```python
from build123d import *

# Parameters (mm, degrees)
BOSS_EXTRUDE1_DEPTH = 1
SKETCH3_W           = 55.6
SKETCH3_H           = 0.9
BOSS_EXTRUDE2_DEPTH = 3.24
FILLET1_R           = 1.5
FILLET2_R           = 1.5
FILLET3_R           = 1.5
FILLET4_R           = 1.5
CUT_EXTRUDE2_REACH  = 3
SKETCH5_R           = 1.6


with BuildPart() as part:
    # Sketch1 → Boss-Extrude1 (new body)
    with BuildSketch(Plane(origin=(0, 0, 0), x_dir=(1, 0, 0), z_dir=(0, 1, 0))):
        with BuildLine():
            Line((27.8, -18.75), (-27.8, -18.75))
            ThreePointArc((-27.8, -18.75), (-32.396194078, -16.846194078), (-34.3, -12.25))
            Line((-34.3, -12.25), (-34.3, 12.25))
            ThreePointArc((-34.3, 12.25), (-32.396194078, 16.846194078), (-27.8, 18.75))
            Line((-27.8, 18.75), (27.8, 18.75))
            ThreePointArc((27.8, 18.75), (32.396194078, 16.846194078), (34.3, 12.25))
            Line((34.3, 12.25), (34.3, -12.25))
            ThreePointArc((34.3, -12.25), (32.396194078, -16.846194078), (27.8, -18.75))
        make_face()
    extrude(amount=BOSS_EXTRUDE1_DEPTH)

    # Sketch3 → Boss-Extrude2 (add)
    with BuildSketch(Plane(origin=(0, 1, 0), x_dir=(1, 0, 0), z_dir=(0, 1, 0))):
        with Locations((0, -18.3)):
            Rectangle(SKETCH3_W, SKETCH3_H)
        with Locations((0, 18.3)):
            Rectangle(SKETCH3_W, SKETCH3_H)
    extrude(amount=BOSS_EXTRUDE2_DEPTH)

    # Fillet1
    fillet1_edges = [part.edges().sort_by_distance(p)[0] for p in [
        (-27.8, 4.24, 18.3),
    ]]
    fillet(fillet1_edges, radius=FILLET1_R)

    # Fillet2
    fillet2_edges = [part.edges().sort_by_distance(p)[0] for p in [
        (27.8, 4.24, 18.3),
    ]]
    fillet(fillet2_edges, radius=FILLET2_R)

    # Fillet3
    fillet3_edges = [part.edges().sort_by_distance(p)[0] for p in [
        (27.8, 4.24, -18.3),
    ]]
    fillet(fillet3_edges, radius=FILLET3_R)

    # Fillet4
    fillet4_edges = [part.edges().sort_by_distance(p)[0] for p in [
        (-27.8, 4.24, -18.3),
    ]]
    fillet(fillet4_edges, radius=FILLET4_R)

    # Sketch5 → Cut-Extrude2 (cut, up to next)
    with BuildSketch(Plane(origin=(0, 1, 0), x_dir=(1, 0, 0), z_dir=(0, 1, 0)), mode=Mode.PRIVATE) as cut_extrude2_sk1:
        with Locations((-25.4, -9.4746)):
            Circle(SKETCH5_R)
    cut_extrude2_tool1 = extrude(cut_extrude2_sk1.sketch, amount=-CUT_EXTRUDE2_REACH, mode=Mode.PRIVATE) & part.part
    add(cut_extrude2_tool1.solids().sort_by_distance((-25.4, 1, 9.4746))[0], mode=Mode.SUBTRACT)
    # Sketch5 → Cut-Extrude2 (cut, up to next)
    with BuildSketch(Plane(origin=(0, 1, 0), x_dir=(1, 0, 0), z_dir=(0, 1, 0)), mode=Mode.PRIVATE) as cut_extrude2_sk2:
        with Locations((-15.24, -9.4746)):
            Circle(SKETCH5_R)
    cut_extrude2_tool2 = extrude(cut_extrude2_sk2.sketch, amount=-CUT_EXTRUDE2_REACH, mode=Mode.PRIVATE) & part.part
    add(cut_extrude2_tool2.solids().sort_by_distance((-15.24, 1, 9.4746))[0], mode=Mode.SUBTRACT)
    # Sketch5 → Cut-Extrude2 (cut, up to next)
    with BuildSketch(Plane(origin=(0, 1, 0), x_dir=(1, 0, 0), z_dir=(0, 1, 0)), mode=Mode.PRIVATE) as cut_extrude2_sk3:
        with Locations((-5.08, -9.4746)):
            Circle(SKETCH5_R)
    cut_extrude2_tool3 = extrude(cut_extrude2_sk3.sketch, amount=-CUT_EXTRUDE2_REACH, mode=Mode.PRIVATE) & part.part
    add(cut_extrude2_tool3.solids().sort_by_distance((-5.08, 1, 9.4746))[0], mode=Mode.SUBTRACT)
    # Sketch5 → Cut-Extrude2 (cut, up to next)
    with BuildSketch(Plane(origin=(0, 1, 0), x_dir=(1, 0, 0), z_dir=(0, 1, 0)), mode=Mode.PRIVATE) as cut_extrude2_sk4:
        with Locations((5.08, -9.4746)):
            Circle(SKETCH5_R)
    cut_extrude2_tool4 = extrude(cut_extrude2_sk4.sketch, amount=-CUT_EXTRUDE2_REACH, mode=Mode.PRIVATE) & part.part
    add(cut_extrude2_tool4.solids().sort_by_distance((5.08, 1, 9.4746))[0], mode=Mode.SUBTRACT)
    # Sketch5 → Cut-Extrude2 (cut, up to next)
    with BuildSketch(Plane(origin=(0, 1, 0), x_dir=(1, 0, 0), z_dir=(0, 1, 0)), mode=Mode.PRIVATE) as cut_extrude2_sk5:
        with Locations((15.24, -9.4746)):
            Circle(SKETCH5_R)
    cut_extrude2_tool5 = extrude(cut_extrude2_sk5.sketch, amount=-CUT_EXTRUDE2_REACH, mode=Mode.PRIVATE) & part.part
    add(cut_extrude2_tool5.solids().sort_by_distance((15.24, 1, 9.4746))[0], mode=Mode.SUBTRACT)
    # Sketch5 → Cut-Extrude2 (cut, up to next)
    with BuildSketch(Plane(origin=(0, 1, 0), x_dir=(1, 0, 0), z_dir=(0, 1, 0)), mode=Mode.PRIVATE) as cut_extrude2_sk6:
        with Locations((25.4, -9.4746)):
            Circle(SKETCH5_R)
    cut_extrude2_tool6 = extrude(cut_extrude2_sk6.sketch, amount=-CUT_EXTRUDE2_REACH, mode=Mode.PRIVATE) & part.part
    add(cut_extrude2_tool6.solids().sort_by_distance((25.4, 1, 9.4746))[0], mode=Mode.SUBTRACT)


solid = part.part
```
Part model, mm, in its own coordinate system. A direction names the side the tool comes from. Round coordinates to 2 decimals unless told otherwise and drop trailing zeros. Loops run counter-clockwise (first coordinate to the right, second up) from the corner with the lowest first, then second, coordinate; pieces in that order, holes last.
Item 1: Cut at A-A, the plane x = 15.24. Give the cut face in (y, z), then the cut area to 3 significant figures.
Item 2: 3-axis set-ups, long thin cutter, end or side, ignore diameter. For faces 4 (the face through (0, 3, -17.85)), 5 (the face through (27.37, 3.79, -18.31)): which of +Z, -Z, +X, -X, +Y, -Y reach the whole face in a straight line?
Item 3: Cut at C-C, the plane z = 16. Give the cut face in (x, y).
Item 4: Mould opens along X. For faces 1 (the face through (27.35, 3.81, 18.29)), 2 (the face through (-15.587, 0.507, 11.037)), 3 (the face through (-27.37, 3.79, 18.29)) say: +X half, -X half, draft (parallel to the pull), parting line (faces both ways), or undercut.
Item 5: Drop flat-ended pins along their axis: P1, Ø0.7, axis at y = 2, z = -18, coming from the -X side; P2, Ø5, axis at x = 5.08, z = 9.47, coming from the +Y side. Give the stop position or say it passes through.
Item 6: Drill centre lines: line 1 (Z direction, x = 1.5, y = 2.4); line 2 (Z direction, x = -15.24, y = 0.85); line 3 (Y direction, x = -7, z = -6.5). Where is each one in solid material? Low to high.
Item 7: Cut at B-B, the plane z = -6. Give the cut face in (x, y), then the cut area to 3 significant figures.
A:
1. outline: (0, -18.75) - (4.24, -18.75) - (4.24, -17.85) - (1, -17.85) - (1, 7.87) - (0, 7.87) - close; (0, 11.07) - (1, 11.07) - (1, 17.85) - (4.24, 17.85) - (4.24, 18.75) - (0, 18.75) - close
1. area: 40.1 mm2
2. face 4: +X, -X, +Y
2. face 5: +Z, -Z, +X, +Y
3. outline: (-33.11, 0) - (33.11, 0) - (33.11, 1) - (-33.11, 1) - close
4. face 1: +X half
4. face 2: undercut
4. face 3: -X half
5. P1: stops at x = -27.8
5. P2: stops at y = 1
6. line 1: z = -18.75 to -17.85, 17.85 to 18.75
6. line 2: z = -18.75 to 7.87, 11.07 to 18.75
6. line 3: y = 0 to 1
7. outline: (-34.3, 0) - (34.3, 0) - (34.3, 1) - (-34.3, 1) - close
7. area: 68.6 mm2
